from build123d import *

# Parameters (mm, degrees)
F0_W     = 135
F0_H     = 87.5
F1_DEPTH = 4
F3_DEPTH = 25


with BuildPart() as f1:
    # F0 (on Top) → F1 (new body)
    with BuildSketch(Plane.XY):
        Rectangle(F0_W, F0_H)
    extrude(amount=F1_DEPTH)

    # F2 (on face) → F3 (cut)
    with BuildSketch(Plane.XY.offset(4)):
        with BuildLine():
            Line((-55, -32.749999), (55, -32.749999))
            ThreePointArc((55, -32.749999), (58.999999, -28.75), (55, -24.750001))
            Line((55, -24.750001), (-55, -24.750001))
            ThreePointArc((-55, -24.750001), (-58.999999, -28.75), (-55, -32.749999))
        make_face()
    extrude(amount=-F3_DEPTH, mode=Mode.SUBTRACT)


solid = f1.part
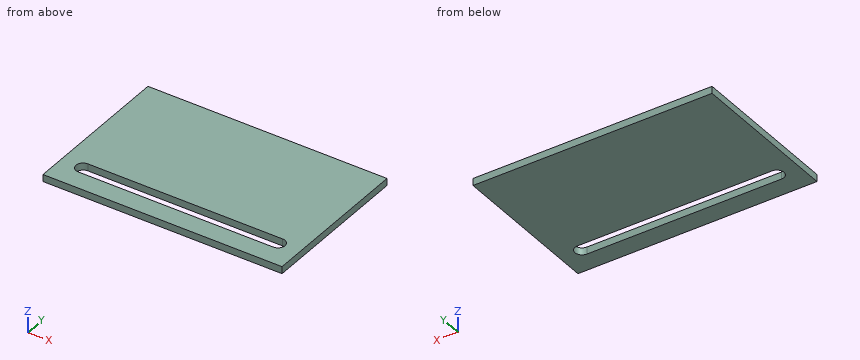
Input: part model. Units: mm. Frame: model coordinates. Coordinates: 2 decimals unless noted, no trailing zeros. Loops run counter-clockwise (first coordinate to the right, second up) from the corner with the lowest first, then second, coordinate; pieces in that order, holes last.
Q1. Cut plane A-A (y = -28.75). Output: boundary loops of the cut face in (x, z), then the cut area to 3 significant figures.
Q2. Cut plane C-C (z = 3.35). Output: boundary loops of the cut face in (x, y), then the cut area to 3 significant figures.
Q3. Material intervals for line 1 (Y direction, x = -49.5, z = 2.8); line 2 (X direction, y = -32, z = 3.85), sorted ascending.
Q4. Cut plane B-B (x = 14.5). Output: boundary loops of the cut face in (y, z).
Working result:
1. outline: (-67.5, 0) - (-59, 0) - (-59, 4) - (-67.5, 4) - close; (59, 0) - (67.5, 0) - (67.5, 4) - (59, 4) - close
1. area: 68.0 mm2
2. outline: (-67.5, -43.75) - (67.5, -43.75) - (67.5, 43.75) - (-67.5, 43.75) - close; hole (-55, -32.75) - (55, -32.75) arc R4 ccw to (55, -24.75) - (-55, -24.75) arc R4 ccw to start
2. area: 10,900 mm2
3. line 1: y = -43.75 to -32.75, -24.75 to 43.75
3. line 2: x = -67.5 to -57.33, 57.33 to 67.5
4. outline: (-43.75, 0) - (-32.75, 0) - (-32.75, 4) - (-43.75, 4) - close; (-24.75, 0) - (43.75, 0) - (43.75, 4) - (-24.75, 4) - close
